Model file for the job. Use its own axes, mm. A direction names the side the tool comes from. Round coordinates to 2 decimals unless told otherwise and drop trailing zeros. Loops run counter-clockwise (first coordinate to the right, second up) from the corner with the lowest first, then second, coordinate; pieces in that order, holes last. Notation, with made-up numbers: M 4,-6 L 52,-6 A17 cw 52,3 Z; hole C -9,44 d5. An arc over 180 degrees is marked long. Use a Markdown table: item, result. Add a question column.
Item 1: Tool access for faces 1 (the cylindrical face through (14.621, 14.09, -14.555)), 2 (the cylindrical face through (19.524, 0.185, 19.555)), 3 (the flat face through (5, 40.95, -3)), 4 (the cylindrical face through (-24.25, 14.78, -0.24)): list every direction of +Z, -Z, +X, -X, +Y, -Y with a clear straight run to the whole face (end or side of a thin tool).
Item 2: Wall check: L1, parallel to X at y = 11.25, z = -16.25 (3 decimals); L2, parallel to Z at x = 15.5, y = 9.5 (3 decimals); L3, parallel to Z at x = 16, y = 10 (3 decimals). Give the ranges that are in metal, low to high. Write a range as from..to.
Item 3: Pin check, flat tips, straight feed: P1, Ø8, axis at y = 10.5, z = -11.5, coming from the -X side; P2, Ø2, axis at x = -4.5, z = 21.5, coming from the -Y side; P3, Ø4, axis at x = -7.5, y = 23, coming from the +Z side; P4, Ø1.5, axis at y = -6, z = 6, coming from the -X side (3 decimals). Stop position of each tip, or through.
Item 4: Saw through at A-A on y = 34. Write the cut outline in (x, z), then the cut area to 3 significant figures.
Item 5: Two-plate mould, pull along Y, no slides. Class faces 5 (the flat face through (0, 16.3, 22)), 6 (the cylindrical face through (17.816, 16.053, 3.956)), 7 (the flat face through (2, 23.21, 2)): +Y half, -Y half, draft (parallel to the pull), parting line (faces both ways), or undercut.
```python
from build123d import *

# Parameters (mm, degrees)
BOSS_EXTRUDE1_DEPTH         = 13.21
SKETCH2_R                   = 8.585
BOSS_EXTRUDE2_DEPTH         = 9.63
SKETCH3_W                   = 2.42
SKETCH3_H                   = 8.85
BOSS_EXTRUDE3_DEPTH         = 0.26
CIRPATTERN2_COUNT           = 10
CIRPATTERN1_COUNT           = 2
CIRPATTERN1_ANGLE           = 90
CIRPATTERN1_COPY_1_SKETCH_W = 2.42
CIRPATTERN1_COPY_1_SKETCH_H = 8.85
CIRPATTERN1_COPY_1_DEPTH    = 0.26
CIRPATTERN1_COPY_2_SKETCH_W = 2.42
CIRPATTERN1_COPY_2_SKETCH_H = 8.85
CIRPATTERN1_COPY_2_DEPTH    = 0.26
CUT_EXTRUDE1_REACH          = 60.953
SKETCH7_R                   = 1.05
CUT_EXTRUDE2_DEPTH          = 4


with BuildPart() as part:
    # Sketch1 → Boss-Extrude1 (new, symmetric)
    with BuildSketch(Plane(origin=(0, 0, 0), x_dir=(1, 0, 0), z_dir=(0, 1, 0))):
        with BuildLine():
            Line((18.125, 20.125), (-18.125, 20.125))
            ThreePointArc((-18.125, 20.125), (-19.539213562, 19.539213562), (-20.125, 18.125))
            Line((-20.125, 18.125), (-20.125, -18.125))
            ThreePointArc((-20.125, -18.125), (-19.539213562, -19.539213562), (-18.125, -20.125))
            Line((-18.125, -20.125), (18.125, -20.125))
            ThreePointArc((18.125, -20.125), (19.539213562, -19.539213562), (20.125, -18.125))
            Line((20.125, -18.125), (20.125, 18.125))
            ThreePointArc((20.125, 18.125), (19.539213562, 19.539213562), (18.125, 20.125))
        make_face()
    extrude(amount=BOSS_EXTRUDE1_DEPTH, both=True)

    # Sketch2 → Boss-Extrude2 (add)
    with BuildSketch(Plane(origin=(20.125, 0, 0), x_dir=(0, 0, -1), z_dir=(1, 0, 0))):
        with Locations(Location((0, 3.395, 0), (0, 0, 180))):
            Circle(SKETCH2_R)
    boss_extrude2 = extrude(amount=BOSS_EXTRUDE2_DEPTH)

    # Sketch3 → Boss-Extrude3 (add)
    with BuildSketch(Plane(origin=(29.755, 0, 0), x_dir=(0, 0, -1), z_dir=(1, 0, 0))):
        with Locations((0, -5.795)):
            Rectangle(SKETCH3_W, SKETCH3_H)
    boss_extrude3 = extrude(amount=BOSS_EXTRUDE3_DEPTH)

    # CirPattern2: Boss-Extrude3 ×10 about axis, 7 skipped
    cirpattern2_axis = Axis((0, 3.395, 0), (1, 0, 0))
    add([boss_extrude3.rotate(cirpattern2_axis, i * 360 / CIRPATTERN2_COUNT) for i in range(1, CIRPATTERN2_COUNT) if i not in (2, 3, 4, 5, 6, 7, 8)])

    # CirPattern1: Boss-Extrude2, Boss-Extrude3 ×2 about axis
    cirpattern1_axis = Axis((0, 0, 0), (0, 1, 0))
    add([boss_extrude2.rotate(cirpattern1_axis, i * CIRPATTERN1_ANGLE / (CIRPATTERN1_COUNT - 1)) for i in range(1, CIRPATTERN1_COUNT)])
    add([boss_extrude3.rotate(cirpattern1_axis, i * CIRPATTERN1_ANGLE / (CIRPATTERN1_COUNT - 1)) for i in range(1, CIRPATTERN1_COUNT)])

    # CirPattern1 copy 1 sketch → CirPattern1 copy 1 (add)
    with BuildSketch(Plane(origin=(-1.995530932, 0.648387304, -29.755), x_dir=(-0.8090169943749475, 0.5877852522924731, 2.9203766201002924e-15), z_dir=(0, 0, -1))):
        with Locations((0, -5.795)):
            Rectangle(CIRPATTERN1_COPY_1_SKETCH_W, CIRPATTERN1_COPY_1_SKETCH_H)
    extrude(amount=CIRPATTERN1_COPY_1_DEPTH)

    # CirPattern1 copy 2 sketch → CirPattern1 copy 2 (add)
    with BuildSketch(Plane(origin=(1.995530932, 0.648387304, -29.755), x_dir=(-0.8090169943749473, -0.5877852522924734, 2.920376620100292e-15), z_dir=(0, 0, -1))):
        with Locations((0, -5.795)):
            Rectangle(CIRPATTERN1_COPY_2_SKETCH_W, CIRPATTERN1_COPY_2_SKETCH_H)
    extrude(amount=CIRPATTERN1_COPY_2_DEPTH)

    # Sketch5 → Revolve1 (revolve)
    with BuildSketch(Plane.XY, mode=Mode.PRIVATE) as revolve1_sk:
        Polygon((0, 13.21), (-24.25, 13.21), (-24.25, 16.3), (-21.25, 16.3), (-21.25, 14.49), (-20.25, 14.49), (-20.25, 17.66), (-18.25, 17.66), (-18.25, 14.49), (-16, 14.49), (-16, 16.3), (-14.25, 16.3), (-14.25, 14.49), (-12, 14.49), (-12, 16.3), (-10.25, 16.3), (-10.25, 14.49), (-8, 14.49), (-8, 16.3), (-6.25, 16.3), (-6.25, 14.49), (-4, 14.49), (-4, 18.21), (-2.485, 21.21), (-2.485, 23.21), (-3.5, 23.21), (-5.985, 35.21), (-5.985, 39), (-5.485, 39), (-5.485, 39.75), (-5.985, 39.75), (-5.985, 40.95), (-5.485, 40.95), (-5.485, 41.7), (-5.985, 41.7), (-5.985, 47.06), (-5.485, 47.06), (-5.485, 47.81), (-5.985, 47.81), (-5.985, 49.01), (-5.485, 49.01), (-5.485, 49.76), (-5.985, 49.76), (-5.985, 50.96), (-5.485, 50.96), (-5.485, 51.71), (-5.985, 51.71), (-5.985, 57.21), (0, 57.21), align=None)
    revolve(revolve1_sk.sketch.rotate(Axis((0, 0, 0), (0, 1, 0)), 270), axis=Axis((0, 0, 0), (0, 1, 0)))

    # Cut-Extrude1: up to this face of the body (flat: up to its plane)
    cut_extrude1_end = Plane(part.part.faces().sort_by_distance((-17.994834976, 13.21, 17.994834976))[0])
    # Sketch6 → Cut-Extrude1 (cut, up to the picked face)
    with BuildSketch(Plane(origin=(0, 16.3, 0), x_dir=(1, 0, 0), z_dir=(0, 1, 0)), mode=Mode.PRIVATE) as cut_extrude1_sk1:
        with BuildLine():
            Line((-17.592816716, 14.587612896), (-18.583978831, 15.57877501))
            ThreePointArc((-18.583978831, 15.57877501), (-17.147339444, 17.147339444), (-15.57877501, 18.583978831))
            Line((-15.57877501, 18.583978831), (-14.587612896, 17.592816716))
            ThreePointArc((-14.587612896, 17.592816716), (-14.587612896, 14.587612896), (-17.592816716, 14.587612896))
        make_face()
    cut_extrude1_tool1 = split(extrude(cut_extrude1_sk1.sketch, amount=-CUT_EXTRUDE1_REACH, mode=Mode.PRIVATE), bisect_by=cut_extrude1_end, keep=Keep.BOTH, mode=Mode.PRIVATE)
    # Sketch6 → Cut-Extrude1 (cut, up to the picked face)
    with BuildSketch(Plane(origin=(0, 16.3, 0), x_dir=(1, 0, 0), z_dir=(0, 1, 0)), mode=Mode.PRIVATE) as cut_extrude1_sk2:
        with BuildLine():
            Line((14.587612896, 17.592816716), (15.57877501, 18.583978831))
            ThreePointArc((15.57877501, 18.583978831), (17.147339444, 17.147339444), (18.583978831, 15.57877501))
            Line((18.583978831, 15.57877501), (17.592816716, 14.587612896))
            ThreePointArc((17.592816716, 14.587612896), (14.587612896, 14.587612896), (14.587612896, 17.592816716))
        make_face()
    cut_extrude1_tool2 = split(extrude(cut_extrude1_sk2.sketch, amount=-CUT_EXTRUDE1_REACH, mode=Mode.PRIVATE), bisect_by=cut_extrude1_end, keep=Keep.BOTH, mode=Mode.PRIVATE)
    # Sketch6 → Cut-Extrude1 (cut, up to the picked face)
    with BuildSketch(Plane(origin=(0, 16.3, 0), x_dir=(1, 0, 0), z_dir=(0, 1, 0)), mode=Mode.PRIVATE) as cut_extrude1_sk3:
        with BuildLine():
            Line((17.592816716, -14.587612896), (18.583978831, -15.57877501))
            ThreePointArc((18.583978831, -15.57877501), (17.147339444, -17.147339444), (15.57877501, -18.583978831))
            Line((15.57877501, -18.583978831), (14.587612896, -17.592816716))
            ThreePointArc((14.587612896, -17.592816716), (14.587612896, -14.587612896), (17.592816716, -14.587612896))
        make_face()
    cut_extrude1_tool3 = split(extrude(cut_extrude1_sk3.sketch, amount=-CUT_EXTRUDE1_REACH, mode=Mode.PRIVATE), bisect_by=cut_extrude1_end, keep=Keep.BOTH, mode=Mode.PRIVATE)
    # Sketch6 → Cut-Extrude1 (cut, up to the picked face)
    with BuildSketch(Plane(origin=(0, 16.3, 0), x_dir=(1, 0, 0), z_dir=(0, 1, 0)), mode=Mode.PRIVATE) as cut_extrude1_sk4:
        with BuildLine():
            Line((-14.587612896, -17.592816716), (-15.57877501, -18.583978831))
            ThreePointArc((-15.57877501, -18.583978831), (-17.147339444, -17.147339444), (-18.583978831, -15.57877501))
            Line((-18.583978831, -15.57877501), (-17.592816716, -14.587612896))
            ThreePointArc((-17.592816716, -14.587612896), (-14.587612896, -14.587612896), (-14.587612896, -17.592816716))
        make_face()
    cut_extrude1_tool4 = split(extrude(cut_extrude1_sk4.sketch, amount=-CUT_EXTRUDE1_REACH, mode=Mode.PRIVATE), bisect_by=cut_extrude1_end, keep=Keep.BOTH, mode=Mode.PRIVATE)
    add(cut_extrude1_tool1.solids().sort_by(Axis((-15.992422, 16.3, -15.992422), (0, -1, 0)))[0], mode=Mode.SUBTRACT)
    add(cut_extrude1_tool2.solids().sort_by(Axis((15.992422, 16.3, -15.992422), (0, -1, 0)))[0], mode=Mode.SUBTRACT)
    add(cut_extrude1_tool3.solids().sort_by(Axis((15.992422, 16.3, 15.992422), (0, -1, 0)))[0], mode=Mode.SUBTRACT)
    add(cut_extrude1_tool4.solids().sort_by(Axis((-15.992422, 16.3, 15.992422), (0, -1, 0)))[0], mode=Mode.SUBTRACT)

    # Sketch7 → Cut-Extrude2 (cut)
    with BuildSketch(Plane(origin=(0, 13.21, 0), x_dir=(1, 0, 0), z_dir=(0, 1, 0))):
        with Locations(Location((-16.25, 16.25, 0), (0, 0, 270))):
            Circle(SKETCH7_R)
        with Locations(Location((16.25, 16.25, 0), (0, 0, 270))):
            Circle(SKETCH7_R)
        with Locations(Location((16.25, -16.25, 0), (0, 0, 90))):
            Circle(SKETCH7_R)
        with Locations(Location((-16.25, -16.25, 0), (0, 0, 90))):
            Circle(SKETCH7_R)
    extrude(amount=-CUT_EXTRUDE2_DEPTH, mode=Mode.SUBTRACT)


solid = part.part
```
Entries:
| question | item | result |
|---|---|---|
| 1 | face 1 | +Y |
| 1 | face 2 | +Z, +X, +Y, -Y |
| 1 | face 3 | none |
| 1 | face 4 | -X, +Y |
| 2 | L1 | -20.125..-17.3, -15.2..15.2, 17.3..20.125 |
| 2 | L2 | -20.125..-16.985, -15.515..15.515, 16.985..20.125 |
| 2 | L3 | -20.125..-17.27, -15.23..15.23, 17.27..20.125 |
| 3 | P1 | x = -22.69 |
| 3 | P2 | y = 13.21 |
| 3 | P3 | through |
| 3 | P4 | x = -20.125 |
| 4 | outline | C 0,0 d11.47 |
| 4 | area | 103 mm2 |
| 5 | face 5 | +Y half |
| 5 | face 6 | draft |
| 5 | face 7 | undercut |
